from build123d import *

# Parameters (mm, degrees)
F0_R      = 2.5
F0_R_2    = 2
F1_DEPTH  = 20
F0_R_3    = 3
F2_DEPTH  = 5
F3_DEPTH  = 10
F4_R      = 3
F4_R_2    = 2.5
F5_DEPTH  = 6
F4_R_3    = 1
F6_DEPTH  = 10
F7_SIZE   = 0.5
F9_DEPTH  = 25
F10_DEPTH = 25


with BuildPart() as f1:
    # F0 (on Right) → F1 (new body)
    with BuildSketch(Plane.YZ):
        Circle(F0_R)
        Circle(F0_R_2, mode=Mode.SUBTRACT)
        Circle(F0_R_2)
    extrude(amount=F1_DEPTH)

    # F0 (on Right) → F2 (join)
    with BuildSketch(Plane.YZ):
        Circle(F0_R_3)
        Circle(F0_R, mode=Mode.SUBTRACT)
    extrude(amount=F2_DEPTH)

    # F0 (on Right) → F3 (cut)
    with BuildSketch(Plane.YZ):
        Circle(F0_R_2)
    extrude(amount=F3_DEPTH, mode=Mode.SUBTRACT)

    # F4 (on face) → F5 (join)
    with BuildSketch(Plane.YZ.offset(20)):
        Circle(F4_R)
        Circle(F4_R_2, mode=Mode.SUBTRACT)
    extrude(amount=-F5_DEPTH)

    # F4 (on face) → F6 (cut)
    with BuildSketch(Plane.YZ.offset(20)):
        Circle(F4_R_3)
    extrude(amount=-F6_DEPTH, mode=Mode.SUBTRACT)

    # F7
    f7_edges = [f1.edges().sort_by_distance(p)[0] for p in [
        (20, -3, 0),
        (0, -3, 0),
    ]]
    chamfer(f7_edges, length=F7_SIZE)

    # F8 (on Front) → F9 (cut)
    with BuildSketch(Plane.XZ):
        with BuildLine():
            ThreePointArc((4, 0), (3, 1), (2, 0))
            Line((2, 0), (4, 0))
        make_face()
        with BuildLine():
            Line((4, 0), (2, 0))
            ThreePointArc((2, 0), (3, -1), (4, 0))
        make_face()
        with BuildLine():
            Line((18, 0), (16, 0))
            ThreePointArc((16, 0), (17, -1), (18, 0))
        make_face()
        with BuildLine():
            ThreePointArc((18, 0), (17, 1), (16, 0))
            Line((16, 0), (18, 0))
        make_face()
    extrude(amount=-F9_DEPTH, mode=Mode.SUBTRACT)

    # F8 (on Front) → F10 (cut)
    with BuildSketch(Plane.XZ):
        with BuildLine():
            ThreePointArc((18, 0), (17, 1), (16, 0))
            Line((16, 0), (18, 0))
        make_face()
        with BuildLine():
            Line((18, 0), (16, 0))
            ThreePointArc((16, 0), (17, -1), (18, 0))
        make_face()
        with BuildLine():
            ThreePointArc((4, 0), (3, 1), (2, 0))
            Line((2, 0), (4, 0))
        make_face()
        with BuildLine():
            Line((4, 0), (2, 0))
            ThreePointArc((2, 0), (3, -1), (4, 0))
        make_face()
    extrude(amount=F10_DEPTH, mode=Mode.SUBTRACT)


solid = f1.part
Can you work these out from the model? Positions are in its coordinate system, mm. A direction names the side the tool comes from. Coordinates: 2 decimals unless noted, no trailing zeros. Loops run counter-clockwise (first coordinate to the right, second up) from the corner with the lowest first, then second, coordinate; pieces in that order, holes last. Notation, with made-up numbers: (-22, 70) - (-12, 70) arc R23 cw to (-12, 98) - close; hole circle Ø7 at (35.25, 43.25). An arc over 180 degrees is marked (long way). Answer as a JSON object with one key per item and string values. Group by question number.
Item 1: If we section it at C-C (z = 0): State how many separate pieces and enclosed holes the cut face has, plus the area to 3 significant figures.
Item 2: For pin 1 (3 mm diameter, centred on x = 7, z = -1, fed in from +Y); pin 2 (2.5 mm diameter, centred on x = 17, z = 0, fed in from -Y); pin 3 (2 mm diameter, centred on y = 0.5, z = 0, fed in from -X); pin 4 (1.5 mm diameter, centred on x = 16, y = 1.5, fed in from -Z), each with a flat end and sliding along its axis, tell me the tip position at first contact or that it passes through.
Item 3: If we section it at B-B (x = 6): List the corners of the cut face in (y, z) for me, plus the area to 3 significant figures.
Item 4: If we section it at A-A (x = 3): List the corners of the cut face in (y, z) for me, plus the area to 3 significant figures.
Item 5: If we mould it in two halves opening along Y, with no side actions, what happens to faces 4 (the face through (20, 1, -1)), 5 (the face through (2.72, 2.77, -1.15)), 6 (the face through (14, -1, 0))? For each: released by +Y, released by -Y, zero draft, split by the parting line, or undercut.
Item 6: If we section it at D-D (x = 17.5): List the corners of the cut face in (y, z) for me.
Item 7: If I drill on L1, parallel to Z at x = 19.4, y = 0; L2, parallel to Z at x = 3, y = 2.45; L3, parallel to Y at x = 13.5, z = 0.75, over which ranges is the centre line in solid material (lowest first)? Write a range as from..to.
Item 8: On a 3-axis mill with a long thin cutter (end or side, diameter ignored), from which of +Z, -Z, +X, -X, +Y, -Y can I reach the whole of each face in a straight line? I mean faces 1 (the face through (5, -2, 2)), 2 (the face through (10, 1, -1)), 3 (the face through (3.8, 2.4, 0.6)). Say none if no direction works.
Returned:
{
 "1": {"separate pieces": "6", "enclosed holes": "0", "area": "38.5 mm²"},
 "2": {"pin 1": "stops at y = 2.5", "pin 2": "stops at y = -3", "pin 3": "stops at x = 10", "pin 4": "stops at z = -2.9"},
 "3": {"outline": "circle Ø5 at (0, 0); hole circle Ø4 at (0, 0)", "area": "7.07 mm²"},
 "4": {"outline": "(-2.83, -1) arc R3 ccw to (2.83, -1) - (1.73, -1) arc R2 cw to (-1.73, -1) - close; (-2.83, 1) - (-1.73, 1) arc R2 cw to (1.73, 1) - (2.83, 1) arc R3 ccw to start", "area": "11.6 mm²"},
 "5": {"face 4": "zero draft", "face 5": "split by the parting line", "face 6": "undercut"},
 "6": {"outline": "(-2.87, -0.87) arc R3 ccw to (2.87, -0.87) - (0.5, -0.87) arc R1 cw to (-0.5, -0.87) - close; (-2.87, 0.87) - (-0.5, 0.87) arc R1 cw to (0.5, 0.87) - (2.87, 0.87) arc R3 ccw to start"},
 "7": {"L1": "z = -3..-1, 1..3", "L2": "z = -1.73..-1, 1..1.73", "L3": "y = -2.38..-0.66, 0.66..2.38"},
 "8": {"face 1": "none", "face 2": "-X", "face 3": "+Y, -Y"}
}
